Autodesk Inventor part; units mm, degrees
ref_plane "YZ Plane" through (0, 0, 0) normal (1, 0, 0) x (0, 1, 0)
ref_plane "XZ Plane" through (0, 0, 0) normal (0, 1, 0) x (-1, 0, 0)
ref_plane "XY Plane" through (0, 0, 0) normal (0, 0, 1) x (1, 0, 0)
sketch "Szkic1" plane through (0, 0, 0) normal (0, 0, 1) x (1, 0, 0)
  line L0 (-7.8594, 6.1623) -> (18.1406, 6.1623)
  line L1 (18.1406, 6.1623) -> (18.1406, -8.8377)
  line L2 (18.1406, -8.8377) -> (-7.8594, -8.8377)
  line L3 (-7.8594, -8.8377) -> (-7.8594, 6.1623)
  point P0 (0, 0)
  point P1 (-2.8594, -1.3377)
  point P2 (13.1406, -1.3377)
  dimension "d0" = 26
  dimension "d1" = 15
  dimension "d4" = 7.5
  dimension "d5" = 7.5
  dimension "d6" = 5
  dimension "d7" = 5
extrude "Wyciągnięcie proste1" add sketch "Szkic1" along normal blind 18
hole "Otwór1" at (-2.8594, -1.3377, 0) at (13.1406, -1.3377, 0) direction (0, 0, 1) diameter 3.1 end through all
sketch "Szkic2" plane through (-7.8594, -8.8377, 0) normal (0, -1, 0) x (1, 0, 0)
  line L0 (26, 0) -> (0, 0)
  line L1 (26, 0) -> (26, 18)
  line L2 (0, 18) -> (26, 18)
  line L3 (0, 0) -> (0, 18)
  point P0 (7.8594, 0)
  point P1 (13, 12)
  point P2 (13, 4)
  dimension "d16" = 8
  dimension "d17" = 13
  dimension "d18" = 26
  dimension "d19" = 13
  dimension "d27" = 4
hole "Otwór2" at (5.1406, -8.8377, 12) at (5.1406, -8.8377, 4) direction (0, 1, 0) diameter 3.1 end through all
chamfer "Faza2" distance 2 angle 45 2 edges at (-7.8594, -8.8377, 9) (18.1406, -8.8377, 9)
sketch "Szkic4" plane through (-5.8594, -8.8377, 0) normal (0, -1, 0) x (1, 0, 0)
  line L0 (22, 18) -> (22, 0)
  line L1 (0, 18) -> (22, 18)
  line L2 (0, 0) -> (0, 18)
  line L3 (22, 0) -> (0, 0)
  circle A0 centre (11, 12) radius 1.55
  circle A1 centre (11, 4) radius 1.55
  line L4 (12.6599, 14.875) -> (14.3198, 12)
  line L5 (14.3198, 12) -> (12.6599, 9.125)
  line L6 (12.6599, 9.125) -> (9.3401, 9.125)
  line L7 (9.3401, 9.125) -> (7.6802, 12)
  line L8 (7.6802, 12) -> (9.3401, 14.875)
  line L9 (9.3401, 14.875) -> (12.6599, 14.875)
  line L10 (12.6599, 6.875) -> (14.3198, 4)
  line L11 (14.3198, 4) -> (12.6599, 1.125)
  line L12 (12.6599, 1.125) -> (9.3401, 1.125)
  line L13 (9.3401, 1.125) -> (7.6802, 4)
  line L14 (7.6802, 4) -> (9.3401, 6.875)
  line L15 (9.3401, 6.875) -> (12.6599, 6.875)
  point P0 (5.8594, 0)
  point P1 (11, 14.875)
  point P2 (11, 6.875)
extrude "Wyciągnięcie proste3" cut sketch "Szkic4" against normal blind 2.5 contours L4 L5 L6 L7 L8 L9 | L10 L11 L12 L13 L14 L15
properties part number "3DP_ABS_Z_Axis_IGUS_Cable_Chain_Mount"
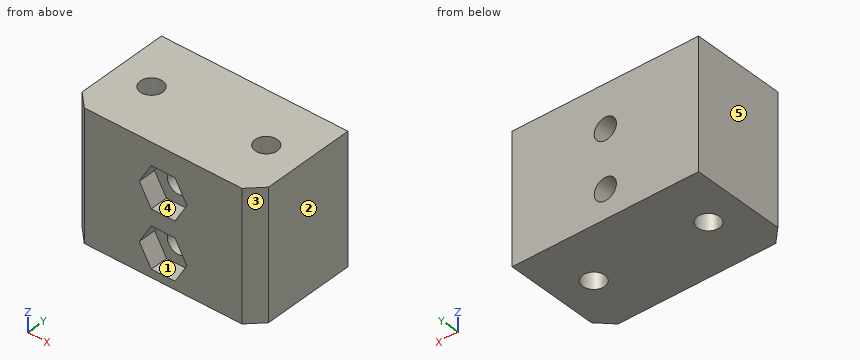
The model under review builds one solid part; all positions refer to its coordinate system, in mm. Face numbers are marked on the shaded views. A direction names the side the tool comes from. Round coordinates to 2 decimals unless told otherwise and drop trailing zeros. Loops run counter-clockwise (first coordinate to the right, second up) from the corner with the lowest first, then second, coordinate; pieces in that order, holes last.
Item 1: For line 1 (Z direction, x = 5, y = -8) (3 decimals); line 2 (Y direction, x = 13.25, z = 13.25); line 3 (X direction, y = -2.5, z = 13.75), list the stretches that pass through material, from the lowest coordinate up.
Determined:
line 1: z = 0 to 1.125, 6.875 to 9.125, 14.875 to 18
line 2: y = -8.84 to -2.88, 0.21 to 6.16
line 3: x = -7.86 to -3.88, -1.83 to 12.12, 14.17 to 18.14
Item 2: For the marked faces 1 and 2, list the 3-axis set-ups (+Z, -Z, +X, -X, +Y, -Y) from which the entire face can be reached by the end or side of a thin tool; tool diameter is ignored.
Determined:
face 1: -Y
face 2: +Z, -Z, +X, +Y, -Y
Item 3: Take a section at C-C (x = 6.25). Write out the cut boundary in (y, z) (3 decimals), then the cut area to 3 significant figures.
Determined:
outline: (-8.838, 0) - (6.162, 0) - (6.162, 2.918) - (-6.338, 2.918) - (-6.338, 1.125) - (-8.838, 1.125) - close; (-8.838, 6.875) - (-6.338, 6.875) - (-6.338, 5.082) - (6.162, 5.082) - (6.162, 10.918) - (-6.338, 10.918) - (-6.338, 9.125) - (-8.838, 9.125) - close; (-8.838, 14.875) - (-6.338, 14.875) - (-6.338, 13.082) - (6.162, 13.082) - (6.162, 18) - (-8.838, 18) - close
area: 187 mm2
Item 4: Mouldability with a two-part tool opening along X and no side actions: class the marked faces 3, 4 and 5 as released by +X, released by -X, zero draft, split by the parting line, or undercut.
Determined:
face 3: released by +X
face 4: undercut
face 5: released by -X
Item 5: Take a section at B-B (x = -3.25). Write out the cut boundary in (y, z).
Determined:
outline: (-8.84, 0) - (-2.84, 0) - (-2.84, 18) - (-8.84, 18) - close; (0.16, 0) - (6.16, 0) - (6.16, 18) - (0.16, 18) - close
Item 6: Take a section at A-A (z = 12.5). Write out the cut boundary in (x, y), then the cut area to 3 significant figures.
Determined:
outline: (-7.86, -6.84) - (-5.86, -8.84) - (2.11, -8.84) - (2.11, -6.34) - (3.67, -6.34) - (3.67, 6.16) - (-7.86, 6.16) - close; (6.61, -6.34) - (8.17, -6.34) - (8.17, -8.84) - (16.14, -8.84) - (18.14, -6.84) - (18.14, 6.16) - (6.61, 6.16) - close; hole circle Ø3.1 at (-2.86, -1.34); hole circle Ø3.1 at (13.14, -1.34)
area: 319 mm2
Item 7: Take a section at D-D (y = -6). Write out the cut boundary in (x, z), then the cut area to 3 significant figures.
Determined:
outline: (-7.86, 0) - (18.14, 0) - (18.14, 18) - (-7.86, 18) - close; hole circle Ø3.1 at (5.14, 4); hole circle Ø3.1 at (5.14, 12)
area: 453 mm2
